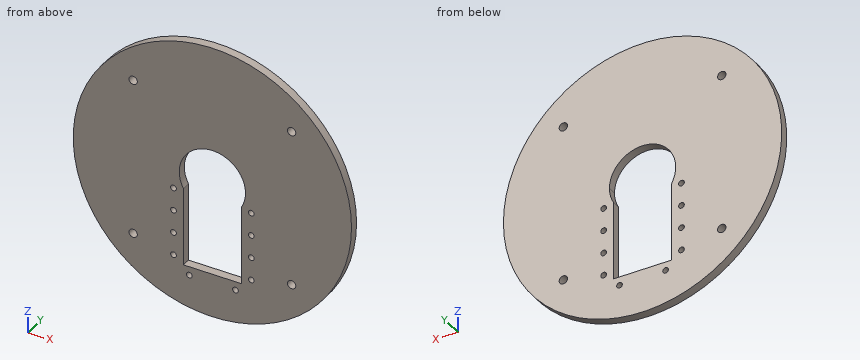
```python
from build123d import *

# Parameters (mm, degrees)
F0_R     = 48.3
F1_DEPTH = 3
F2_R     = 1.25
F2_R_2   = 2.5
F3_DEPTH = 3.001
F4_R     = 1.45
F5_DEPTH = 3.001
F6_R     = 1
F7_DEPTH = 3.001


with BuildPart() as f1:
    # F0 (on Front) → F1 (new body)
    with BuildSketch(Plane.XZ):
        Circle(F0_R)
    extrude(amount=F1_DEPTH)

    # F2 (on face) → F3 (cut, through all)
    with BuildSketch(Plane.XZ.offset(3)):
        with Locations((-8, 0)):
            Circle(F2_R)
        with Locations((8, 0)):
            Circle(F2_R)
        Circle(F2_R_2)
    extrude(amount=-F3_DEPTH, mode=Mode.SUBTRACT)

    # F4 (on face) → F5 (cut, through all)
    with BuildSketch(Plane.XZ.offset(3)):
        with Locations((-27.5, 27.5)):
            Circle(F4_R)
        with Locations((27.5, 27.5)):
            Circle(F4_R)
        with Locations((-27.5, -27.5)):
            Circle(F4_R)
        with Locations((27.5, -27.5)):
            Circle(F4_R)
    extrude(amount=-F5_DEPTH, mode=Mode.SUBTRACT)

    # F6 (on face) → F7 (cut, through all)
    with BuildSketch(Plane.XZ.offset(3)):
        with BuildLine():
            Line((-10.05, -33), (10.05, -33))
            Line((10.05, -33), (10.05, -5.5899463325))
            ThreePointArc((10.05, -5.5899463325), (0, -11.5), (-10.05, -5.5899463325))
            Line((-10.05, -5.5899463325), (-10.05, -33))
        make_face()
        with BuildLine():
            ThreePointArc((-10.05, -5.5899463325), (0, -11.5), (10.05, -5.5899463325))
            Line((10.05, -5.5899463325), (10.05, 0))
            Line((10.05, 0), (-10.05, 0))
            Line((-10.05, 0), (-10.05, -5.5899463325))
        make_face()
        with BuildLine():
            Line((10.05, 0), (10.05, -5.5899463325))
            ThreePointArc((10.05, -5.5899463325), (11.1315991663, -2.8874729436), (11.5, 0))
            ThreePointArc((11.5, 0), (-2.8874729436, 11.1315991663), (-10.05, -5.5899463325))
            Line((-10.05, -5.5899463325), (-10.05, 0))
            Line((-10.05, 0), (10.05, 0))
        make_face()
        with Locations((-13.5, -6.5)):
            Circle(F6_R)
        with Locations((-13.5, -14.5)):
            Circle(F6_R)
        with Locations((-13.5, -22.5)):
            Circle(F6_R)
        with Locations((-13.5, -30.5)):
            Circle(F6_R)
        with Locations((13.5, -6.5)):
            Circle(F6_R)
        with Locations((13.5, -14.5)):
            Circle(F6_R)
        with Locations((13.5, -22.5)):
            Circle(F6_R)
        with Locations((13.5, -30.5)):
            Circle(F6_R)
        with Locations((-8, -36)):
            Circle(F6_R)
        with Locations((8, -36)):
            Circle(F6_R)
    extrude(amount=-F7_DEPTH, mode=Mode.SUBTRACT)


solid = f1.part
```
Input: part model. Units: mm. Frame: model coordinates. Coordinates: 2 decimals unless noted, no trailing zeros. Order: outer loops, then holes, each group sorted by start corner. A loop starts at its lowest first (then second) coordinate and runs counter-clockwise, first axis right, second up. Notation, with made-up numbers: (55, 6) - (109, 6) arc R21 cw to (109, 32) - close; hole circle Ø7 at (62.5, 36.25). An arc over 180 degrees is marked (long way). Put each result on its own line as item: value.
1. Cut plane C-C on y = -0.6. State how many separate pieces and enclosed holes the cut face has, then the cut area to 3 significant figures.
Report:
separate pieces: 1
enclosed holes: 15
area: 6,390 mm2
2. Cut plane B-B on z = -3. Return the cut outline in (x, y), then the cut area to 3 significant figures.
Report:
outline: (-48.21, -3) - (-11.1, -3) - (-11.1, 0) - (-48.21, 0) - close; (11.1, -3) - (48.21, -3) - (48.21, 0) - (11.1, 0) - close
area: 223 mm2
3. Contact query for flat-ended pins moving along their axis: pin 1 Ø1.5 at (y, z) = (-1, -25.5) entering from +X; pin 2 Ø0.9 at (x, y) = (2, -1) entering from +Z; pin 3 Ø1 at (x, y) = (13, -2.5) entering from +Z. Output: stop coordinate, or through.
Report:
pin 1: stops at x = 41.48
pin 2: stops at z = 48.28
pin 3: stops at z = 46.65
4. Cut plane A-A on x = 0. Return the cut outline in (y, z), then the cut area to 3 significant figures.
Report:
outline: (-3, -48.3) - (0, -48.3) - (0, -33) - (-3, -33) - close; (-3, 11.5) - (0, 11.5) - (0, 48.3) - (-3, 48.3) - close
area: 156 mm2
5. Cut plane D-D on z = 27.5. Return the cut outline in (x, y).
Report:
outline: (-39.71, -3) - (-28.95, -3) - (-28.95, 0) - (-39.71, 0) - close; (-26.05, -3) - (26.05, -3) - (26.05, 0) - (-26.05, 0) - close; (28.95, -3) - (39.71, -3) - (39.71, 0) - (28.95, 0) - close
6. Line query: line 1 along Z through (x, y) = (-13.5, -1.25) (3 decimals); line 2 along Z through (x, y) = (-28, -2.4); line 3 along Z through (x, y) = (-27.5, -2.05). Output: solid intervals per line, ascending.
Report:
line 1: z = -46.375 to -31.5, -29.5 to -23.5, -21.5 to -15.5, -13.5 to -7.5, -5.5 to 46.375
line 2: z = -39.36 to -28.86, -26.14 to 26.14, 28.86 to 39.36
line 3: z = -39.71 to -28.95, -26.05 to 26.05, 28.95 to 39.71
